Can you work these out from the model? Positions are in its coordinate system, mm. A direction names the side the tool comes from. Give positions to 0.01 mm unless a question says otherwise; leave off trailing zeros. Order: outer loops, then holes, each group sorted by start corner. A loop starts at its lowest first (then second) coordinate and runs counter-clockwise, first axis right, second up. Notation, with made-up numbers: (2, 5.25) - (41, 5.25) arc R26 ccw to (41, 37.25) - close; hole circle Ø5 at (65.25, 79). An arc over 180 degrees is marked (long way). Answer as a JSON object with one key per item and string values.
```python
from build123d import *

# Parameters (mm, degrees)
SKETCH_2_W               = 240.549430728
SKETCH_2_H               = 149.540933388
EXTRUDE_1_DEPTH          = 5
SKETCH_6_W               = 93.246571425
SKETCH_6_H               = 149.540933388
EXTRUDE_4_DEPTH          = 5
SKETCH_8_W               = 274.716709757
SKETCH_8_H               = 58.51354913
EXTRUDE_6_DEPTH          = 5
CUT_EXTRUDE_2_DEPTH      = 252.755772101
CUT_EXTRUDE_2_DEPTH_BACK = 252.755772101
SKETCH_9_W               = 59.079292396
SKETCH_9_H               = 149.540933388
SKETCH_10_W              = 104.703380117
SKETCH_10_H              = 208.054482518
CUT_EXTRUDE_3_DEPTH      = 10
SKETCH_12_W              = 200
SKETCH_12_H              = 200
EXTRUDE_7_DEPTH          = 5
SKETCH_13_OUTSIDE_W      = 259.728
SKETCH_13_OUTSIDE_H      = 267.782
SKETCH_13_OUTSIDE_W_2    = 200
SKETCH_13_OUTSIDE_H_2    = 200
CUT_EXTRUDE_4_DEPTH      = 278.64321362
EXTRUDE_START            = -75
SKETCH_18_R              = 5.25
EXTRUDE_9_DEPTH          = 10
EXTRUDE_START_2          = -46
EXTRUDE_10_DEPTH         = 15
EXTRUDE_START_3          = -91.2
EXTRUDE_11_DEPTH         = 15
EXTRUDE_12_REACH         = 307.894
SKETCH_20_R              = 5.25
SKETCH_26_W              = 200
SKETCH_26_H              = 5
EXTRUDE_13_DEPTH         = 100
SKETCH_27_W              = 200
SKETCH_27_H              = 5
CUT_EXTRUDE_5_DEPTH      = 30
EXTRUDE_14_DEPTH         = 10
SKETCH_29_W              = 60
SKETCH_29_H              = 9
EXTRUDE_15_DEPTH         = 10
HOLE_WIZARD_M4_1_D       = 3.3
HOLE_WIZARD_M4_2_D       = 3.3
HOLE_WIZARD_M4_3_D       = 3.3
EXTRUDE_16_DEPTH         = 10
SKETCH_37_W              = 60
SKETCH_37_H              = 9
EXTRUDE_17_DEPTH         = 10
HOLE_WIZARD_M4_4_D       = 3.3
EXTRUDE_START_4          = -3.5
SKETCH_40_R              = 5.25
SKETCH_40_R_2            = 3.25
EXTRUDE_18_DEPTH         = 46.5
CUT_EXTRUDE_START        = -3.5
SKETCH_41_R              = 5.25
SKETCH_41_R_2            = 3.25
CUT_EXTRUDE_6_DEPTH      = 3.5
HOLE_WIZARD_M4_5_D       = 3.3
SKETCH_44_W              = 270
SKETCH_44_H              = 5
CUT_EXTRUDE_7_DEPTH      = 400.170489639
CUT_EXTRUDE_8_DEPTH      = 274.053696703
CUT_EXTRUDE_8_DEPTH_BACK = 274.053696703
SKETCH_45_W              = 100.422934587
SKETCH_45_H              = 170.865744653


with BuildPart() as part:
    # 草图2 → 凸台-拉伸1 (new body)
    with BuildSketch(Plane(origin=(0, 0, 0), x_dir=(1, 0, 0), z_dir=(0, 1, 0))):
        Rectangle(SKETCH_2_W, SKETCH_2_H)
    extrude(amount=EXTRUDE_1_DEPTH)

    # 草图6 → 凸台-拉伸4 (add)
    with BuildSketch(Plane(origin=(0, 5, 0), x_dir=(1, 0, 0), z_dir=(0, 1, 0))):
        with Locations((166.898001077, 0)):
            Rectangle(SKETCH_6_W, SKETCH_6_H)
    extrude(amount=-EXTRUDE_4_DEPTH)

    # 草图8 → 凸台-拉伸6 (add)
    with BuildSketch(Plane(origin=(0, 5, 0), x_dir=(1, 0, 0), z_dir=(0, 1, 0))):
        with Locations((76.162931911, -104.027241259)):
            Rectangle(SKETCH_8_W, SKETCH_8_H)
    extrude(amount=-EXTRUDE_6_DEPTH)

    # 草图9 → 切除-拉伸2 (cut, two sides: drawn at the far end of the back side and taken through both)
    with BuildSketch(Plane(origin=(0, 5, 0), x_dir=(1, 0, 0), z_dir=(0, 1, 0)).offset(-CUT_EXTRUDE_2_DEPTH_BACK)):
        with Locations((-90.735069166, 0)):
            Rectangle(SKETCH_9_W, SKETCH_9_H)
    extrude(amount=CUT_EXTRUDE_2_DEPTH + CUT_EXTRUDE_2_DEPTH_BACK, mode=Mode.SUBTRACT)

    # 草图10 → 切除-拉伸3 (cut)
    with BuildSketch(Plane(origin=(0, 5, 0), x_dir=(1, 0, 0), z_dir=(0, 1, 0))):
        with Locations((-8.84373291, -29.256774565)):
            Rectangle(SKETCH_10_W, SKETCH_10_H)
    extrude(amount=-CUT_EXTRUDE_3_DEPTH, mode=Mode.SUBTRACT)

    # 草图12 → 凸台-拉伸7 (add)
    with BuildSketch(Plane(origin=(0, 5, 0), x_dir=(1, 0, 0), z_dir=(0, 1, 0))):
        with Locations((143.507957149, -25.229533306)):
            Rectangle(SKETCH_12_W, SKETCH_12_H)
    extrude(amount=-EXTRUDE_7_DEPTH)

    # 草图13 outside → 切除-拉伸4 (cut, through all)
    with BuildSketch(Plane(origin=(0, 5, 0), x_dir=(1, 0, 0), z_dir=(0, 1, 0))):
        with Locations((143.508, -29.257)):
            Rectangle(SKETCH_13_OUTSIDE_W, SKETCH_13_OUTSIDE_H)
        with Locations((143.507957149, -25.229533306)):
            Rectangle(SKETCH_13_OUTSIDE_W_2, SKETCH_13_OUTSIDE_H_2, mode=Mode.SUBTRACT)
    extrude(amount=-CUT_EXTRUDE_4_DEPTH, mode=Mode.SUBTRACT)

    # 草图18 → 凸台-拉伸9 (add)
    with BuildSketch(Plane.XY.offset(125.229533306).offset(EXTRUDE_START)):
        with BuildLine():
            Line((95.507957149, 14), (95.507957149, 125))
            ThreePointArc((95.507957149, 125), (88.507957149, 132), (81.507957149, 125))
            Line((81.507957149, 125), (81.507957149, 14))
            Line((81.507957149, 14), (68.507957149, 14))
            Line((68.507957149, 14), (68.507957149, 5))
            Line((68.507957149, 5), (108.507957149, 5))
            Line((108.507957149, 5), (108.507957149, 14))
            Line((108.507957149, 14), (95.507957149, 14))
        make_face()
        with Locations((88.507957149, 125)):
            Circle(SKETCH_18_R, mode=Mode.SUBTRACT)
    extrude_9 = extrude(amount=-EXTRUDE_9_DEPTH)

    # 镜向1: 凸台-拉伸9 across plane
    add(extrude_9.mirror(Plane.XY.offset(25.229533306)))

    # 草图16 → 凸台-拉伸10 (add)
    with BuildSketch(Plane(origin=(243.507957149, 0, 0), x_dir=(0, 0, -1), z_dir=(1, 0, 0)).offset(EXTRUDE_START_2)):
        with BuildLine():
            Line((-53.779533306, 14), (-53.779533306, 145.085631965))
            Line((-53.779533306, 145.085631965), (-67.779533306, 145.085631965))
            Line((-67.779533306, 145.085631965), (-67.779533306, 139.085631965))
            ThreePointArc((-67.779533306, 139.085631965), (-69.779533306, 114.75), (-71.779533306, 139.085631965))
            Line((-71.779533306, 139.085631965), (-71.779533306, 145.085631965))
            Line((-71.779533306, 145.085631965), (-85.779533306, 145.085631965))
            Line((-85.779533306, 145.085631965), (-85.779533306, 14))
            Line((-85.779533306, 14), (-99.779533306, 14))
            Line((-99.779533306, 14), (-99.779533306, 5))
            Line((-99.779533306, 5), (-39.779533306, 5))
            Line((-39.779533306, 5), (-39.779533306, 14))
            Line((-39.779533306, 14), (-53.779533306, 14))
        make_face()
    extrude(amount=-EXTRUDE_10_DEPTH)

    # 草图19 → 凸台-拉伸11 (add)
    with BuildSketch(Plane(origin=(243.507957149, 0, 0), x_dir=(0, 0, -1), z_dir=(1, 0, 0)).offset(EXTRUDE_START_3)):
        with BuildLine():
            Line((37.990466694, 14), (37.990466694, 144.933566106))
            Line((37.990466694, 144.933566106), (23.990466694, 144.933566106))
            Line((23.990466694, 144.933566106), (23.990466694, 138.933566106))
            ThreePointArc((23.990466694, 138.933566106), (21.990466694, 114.9), (19.990466694, 138.933566106))
            Line((19.990466694, 138.933566106), (19.990466694, 144.933566106))
            Line((19.990466694, 144.933566106), (5.990466694, 144.933566106))
            Line((5.990466694, 144.933566106), (5.990466694, 14))
            Line((5.990466694, 14), (-8.009533306, 14))
            Line((-8.009533306, 14), (-8.009533306, 5))
            Line((-8.009533306, 5), (51.990466694, 5))
            Line((51.990466694, 5), (51.990466694, 14))
            Line((51.990466694, 14), (37.990466694, 14))
        make_face()
    extrude(amount=-EXTRUDE_11_DEPTH)

    # 草图20 → 凸台-拉伸12 (add, up to next)
    with BuildSketch(Plane(origin=(0, 0, 40.229533306), x_dir=(-1, 0, 0), z_dir=(0, 0, -1)), mode=Mode.PRIVATE) as extrude_12_sk1:
        with BuildLine():
            Line((-108.507957149, 5), (-68.507957149, 5))
            Line((-68.507957149, 5), (-68.507957149, 14))
            Line((-68.507957149, 14), (-81.507957149, 14))
            Line((-81.507957149, 14), (-81.507957149, 125))
            ThreePointArc((-81.507957149, 125), (-88.507957149, 132), (-95.507957149, 125))
            Line((-95.507957149, 125), (-95.507957149, 14))
            Line((-95.507957149, 14), (-108.507957149, 14))
            Line((-108.507957149, 14), (-108.507957149, 5))
        make_face()
        with Locations(Location((-88.507957149, 125, 0), (0, 0, 180))):
            Circle(SKETCH_20_R, mode=Mode.SUBTRACT)
    extrude_12_tool1 = extrude(extrude_12_sk1.sketch, amount=EXTRUDE_12_REACH, mode=Mode.PRIVATE) - part.part
    add(extrude_12_tool1.solids().sort_by_distance((88.507957, 57.997401, 40.229533))[0])

    # 草图26 → 凸台-拉伸13 (add)
    with BuildSketch(Plane(origin=(243.507957149, 0, 0), x_dir=(0, 0, -1), z_dir=(1, 0, 0))):
        with Locations((-25.229533306, 2.5)):
            Rectangle(SKETCH_26_W, SKETCH_26_H)
    extrude(amount=EXTRUDE_13_DEPTH)

    # 草图27 → 切除-拉伸5 (cut)
    with BuildSketch(Plane(origin=(343.507957149, 0, 0), x_dir=(0, 0, -1), z_dir=(1, 0, 0))):
        with Locations((-25.229533306, 2.5)):
            Rectangle(SKETCH_27_W, SKETCH_27_H)
    extrude(amount=-CUT_EXTRUDE_5_DEPTH, mode=Mode.SUBTRACT)

    # 草图28 → 凸台-拉伸14 (add)
    with BuildSketch(Plane(origin=(197.507957149, 0, 0), x_dir=(0, 0, -1), z_dir=(1, 0, 0))):
        Polygon((-85.779533306, 14), (-53.779533306, 14), (-39.779533306, 14), (-39.779533306, 5), (-99.779533306, 5), (-99.779533306, 14), align=None)
    extrude(amount=EXTRUDE_14_DEPTH)

    # 草图29 → 凸台-拉伸15 (add)
    with BuildSketch(Plane.ZY.offset(-182.507957149)):
        with Locations((69.779533306, 9.5)):
            Rectangle(SKETCH_29_W, SKETCH_29_H)
    extrude(amount=EXTRUDE_15_DEPTH)

    # M4 螺纹孔1 (through all)
    with Locations(Plane(origin=(0, 14, 0), x_dir=(1, 0, 0), z_dir=(0, 1, 0))):
        with Locations((178.507957149, -47.779533306), (201.507957149, -47.779533306), (201.507957149, -91.779533306), (178.507957149, -91.779533306)):
            Hole(HOLE_WIZARD_M4_1_D / 2)

    # M4 螺纹孔2 (through all)
    with Locations(Plane.XY.offset(85.779533306)):
        with Locations((190.007957149, 141.085631965)):
            Hole(HOLE_WIZARD_M4_2_D / 2)

    # M4 螺纹孔3 (through all)
    with Locations(Plane.XY.offset(-5.990466694)):
        with Locations((144.807957149, 140.933566106)):
            Hole(HOLE_WIZARD_M4_3_D / 2)

    # 草图36 → 凸台-拉伸16 (add)
    with BuildSketch(Plane(origin=(152.307957149, 0, 0), x_dir=(0, 0, -1), z_dir=(1, 0, 0))):
        Polygon((5.990466694, 14), (37.990466694, 14), (51.990466694, 14), (51.990466694, 5), (-8.009533306, 5), (-8.009533306, 14), align=None)
    extrude(amount=EXTRUDE_16_DEPTH)

    # 草图37 → 凸台-拉伸17 (add)
    with BuildSketch(Plane.ZY.offset(-137.307957149)):
        with Locations((-21.990466694, 9.5)):
            Rectangle(SKETCH_37_W, SKETCH_37_H)
    extrude(amount=EXTRUDE_17_DEPTH)

    # M4 螺纹孔4 (through all)
    with Locations(Plane(origin=(0, 14, 0), x_dir=(1, 0, 0), z_dir=(0, 1, 0))):
        with Locations((133.307957149, 43.990466694), (156.307957149, 43.990466694), (156.307957149, -0.009533306), (133.307957149, -0.009533306)):
            Hole(HOLE_WIZARD_M4_4_D / 2)

    # 草图40 → 凸台-拉伸18 (add)
    with BuildSketch(Plane.XY.offset(50.229533306).offset(EXTRUDE_START_4)):
        with Locations((88.507957149, 125)):
            Circle(SKETCH_40_R)
        with Locations((88.507957149, 125)):
            Circle(SKETCH_40_R_2, mode=Mode.SUBTRACT)
    extrude(amount=-EXTRUDE_18_DEPTH)

    # 草图41 → 切除-拉伸6 (cut)
    with BuildSketch(Plane(origin=(0, 0, 0.229533306), x_dir=(-1, 0, 0), z_dir=(0, 0, -1)).offset(CUT_EXTRUDE_START)):
        with Locations(Location((-88.507957149, 125, 0), (0, 0, 180))):
            Circle(SKETCH_41_R)
        with Locations(Location((-88.507957149, 125, 0), (0, 0, 180))):
            Circle(SKETCH_41_R_2, mode=Mode.SUBTRACT)
    extrude(amount=CUT_EXTRUDE_6_DEPTH, mode=Mode.SUBTRACT)

    # M4 螺纹孔5 (through all)
    with Locations(Plane(origin=(0, 14, 0), x_dir=(1, 0, 0), z_dir=(0, 1, 0))):
        with Locations((73.507957149, -8.229533306), (103.507957149, -8.229533306), (103.507957149, -42.229533306), (73.507957149, -42.229533306)):
            Hole(HOLE_WIZARD_M4_5_D / 2)

    # 草图44 → 切除-拉伸7 (cut, through all)
    with BuildSketch(Plane.XY.offset(125.229533306)):
        with Locations((178.507957149, 2.5)):
            Rectangle(SKETCH_44_W, SKETCH_44_H)
    extrude(amount=-CUT_EXTRUDE_7_DEPTH, mode=Mode.SUBTRACT)


with BuildPart() as cut_extrude_7_piece_1:
    # of the separate pieces the step leaves, piece 1, a body of its own (cut_extrude_7_pieces)
    add(part.part.solids().sort_by_distance((68.507957149, 14, 50.229533306))[0])


with BuildPart() as cut_extrude_7_piece_2:
    # of the separate pieces the step leaves, piece 2, a body of its own (cut_extrude_7_pieces)
    add(part.part.solids().sort_by_distance((127.307957149, 14, 8.009533306))[0])


with BuildPart() as cut_extrude_7_piece_3:
    # of the separate pieces the step leaves, piece 3, a body of its own (cut_extrude_7_pieces)
    add(part.part.solids().sort_by_distance((172.507957149, 14, 99.779533306))[0])


with BuildPart() as cut_extrude_8_tool:
    # 草图45 → 切除-拉伸8 (new, two sides: drawn at the far end of the back side and taken through both)
    with BuildSketch(Plane.XY.offset(50.229533306).offset(-CUT_EXTRUDE_8_DEPTH_BACK)):
        with Locations((168.17278759, 76.071196607)):
            Rectangle(SKETCH_45_W, SKETCH_45_H)
    extrude(amount=CUT_EXTRUDE_8_DEPTH + CUT_EXTRUDE_8_DEPTH_BACK)


with BuildPart() as cut_extrude_7_piece_2_1:
    add(cut_extrude_7_piece_2.part)

    # 切除-拉伸8: cut by cut_extrude_8_tool
    add(cut_extrude_8_tool.part, mode=Mode.SUBTRACT)


with BuildPart() as cut_extrude_7_piece_3_1:
    add(cut_extrude_7_piece_3.part)

    # 切除-拉伸8: cut by cut_extrude_8_tool
    add(cut_extrude_8_tool.part, mode=Mode.SUBTRACT)


solid = cut_extrude_7_piece_1.part
```
Q1. We'd pull the mould along X, two halves only. Please class faces 1 (the face through (75, 14, 26)), 2 (the face through (88.66, 132, 25.58)), 3 (the face through (102, 9.4, 8.9)): released by +X, released by -X, zero draft, split by the parting line, or undercut.
Recorded:
{"face 1": "zero draft", "face 2": "split by the parting line", "face 3": "undercut"}
Q2. Which directions (+Z, -Z, +X, -X, +Y, -Y) give clear straight access to the entire face, cutting with the end or side of a thin tool? Please do faces 4 (the face through (88.4, 128.4, 3.73)), 5 (the face through (81.508, 70, 26)), 6 (the face through (88.4, 121.6, 46.73)).
Recorded:
{"face 4": "-Z", "face 5": "+Z, -Z, -X, +Y", "face 6": "+Z"}
Q3. If we section it at A-A, the plane z = 11.5: Please give me the cut outline in (x, y).
Recorded:
{"outline": "(68.51, 5) - (108.51, 5) - (108.51, 14) - (95.51, 14) - (95.51, 125) arc R7 ccw to (81.51, 125) - (81.51, 14) - (68.51, 14) - close; hole circle Ø6.5 at (88.51, 125)"}
Q4. I need wall thicknesses on L1, parallel to Z at x = 103.5, y = 13; L2, parallel to X at y = 125, z = 24; L3, parallel to X at y = 125, z = 2. Which ranges of each line are inside material? Lowest first, please.
Recorded:
{"L1": "z = 0.23 to 6.58, 9.88 to 40.58, 43.88 to 50.23", "L2": "x = 81.51 to 85.26, 91.76 to 95.51", "L3": "x = 81.51 to 83.26, 93.76 to 95.51"}
Q5. If we section it at C-C, the plane y = 26.5: Please give me the cut outline in (x, z), then the cut area to 3 significant figures.
Recorded:
{"outline": "(81.51, 0.23) - (95.51, 0.23) - (95.51, 50.23) - (81.51, 50.23) - close", "area": "700 mm^2"}
Q6. I'm going to push flat-ended pins straight in: pin 1 Ø4 at (x, z) = (72, 19.5) entering from +Y; pin 2 Ø5 at (x, z) = (97, 40.5) entering from +Y; pin 3 Ø2.5 at (x, z) = (103.51, 8.23) entering from +Y; pin 4 Ø25 at (y, z) = (61, 18) entering from -X. Where does each tip first touch, or does it pass through?
Recorded:
{"pin 1": "stops at y = 14", "pin 2": "stops at y = 128.62", "pin 3": "passes through", "pin 4": "stops at x = 81.51"}
Q7. If we section it at B-B, the plane x = 79.5: Please give me the cut outline in (y, z).
Recorded:
{"outline": "(5, 0.23) - (14, 0.23) - (14, 50.23) - (5, 50.23) - close"}
